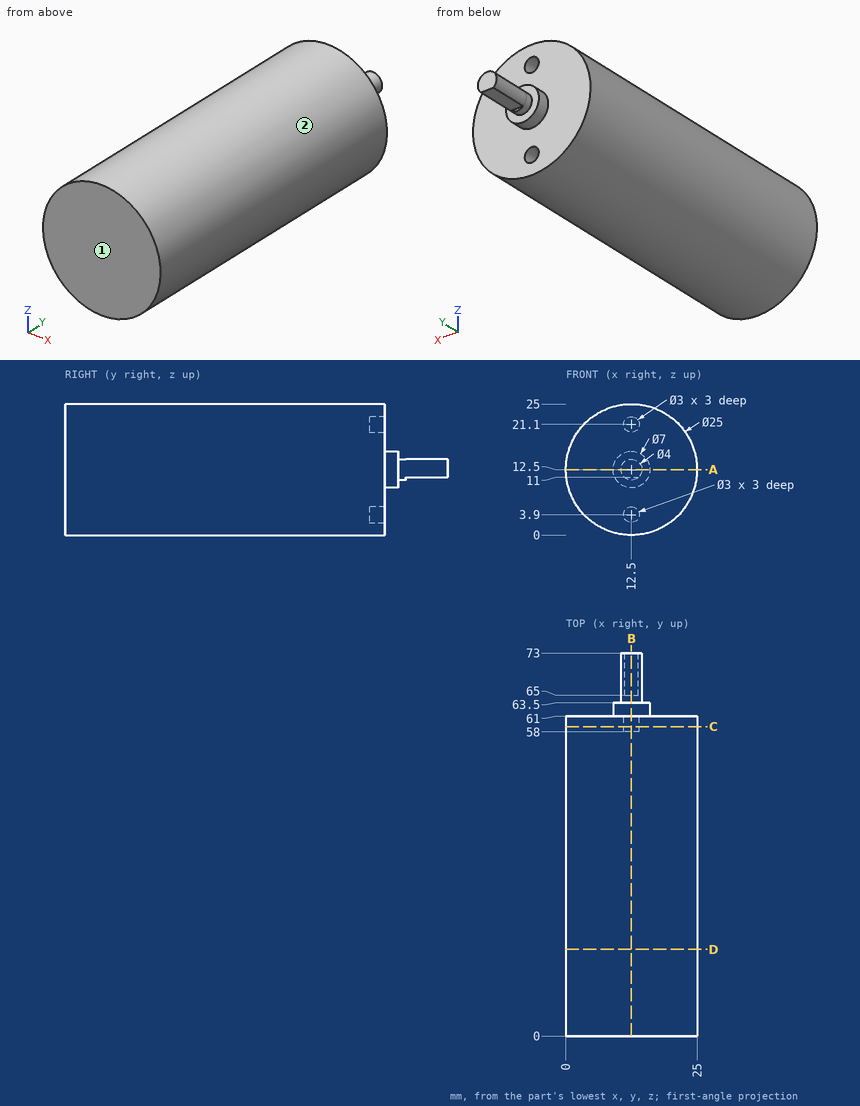
Geometry check sheet. Reference: drawing and pictorial views, mm from the part's lowest x, y, z. Give positions to 0.01 mm unless a question says otherwise; leave off trailing zeros. Loops run counter-clockwise (first coordinate to the right, second up) from the corner with the lowest first, then second, coordinate; pieces in that order, holes last. Notation, with made-up numbers: M 20.5,-1.5 L 34.5,-1.5 A13 cw 34.5,6.5 Z; hole C 37,73 d1. An arc over 180 degrees is marked long. Use a Markdown table: item, result. Add a question column.
Q1. Scan lines: line 1 along Y through (x, z) = (21, 13); line 2 along X through (y, z) = (9, 12.75); line 3 along X through (y, z) = (60.3, 3.9). Record each from-to range of solid material in increasing order. Write a range as [from, to].
Q2. Sectioned sample at C-C, the plane y = 59. Record the cut outline in (x, z).
Q3. Sectioned sample at B-B, the plane x = 12.5. Record the cut outline in (y, z).
Q4. Go/stop test with flat-tipped pins: pin 1 (4 mm diameter, centred on y = 9.5, z = 3.5, fed in from -X); pin 2 (1.5 mm diameter, centred on x = 3.5, y = 45.5, fed in from -Z); pin 3 (0.9 mm diameter, centred on x = 13, z = 3.5, fed in from +Y). Record where each tip stops, or that it passes through.
Q5. Mould release check, pull along X, two halves, no side actions. Record for the marked faces 1 and 2: pulls with the +X half, pulls with the -X half, needs draft (parallel to the pull), parting line crosses it, or undercut.
Q6. Sectioned sample at D-D, the plane y = 16.5. Record the cut outline in (x, z), then the cut area to 3 significant figures.
Q7. Sectioned sample at A-A, the plane z = 12.5. Record the cut outline in (x, y), then the cut area to 3 significant figures.
Verdict:
| question | item | result |
|---|---|---|
| 1 | line 1 | [0, 61] |
| 1 | line 2 | [0, 25] |
| 1 | line 3 | [3.43, 11], [14, 21.57] |
| 2 | outline | C 12.5,12.5 d25; hole C 12.5,3.9 d3; hole C 12.5,21.1 d3 |
| 3 | outline | M 0,0 L 61,0 L 61,2.4 L 58,2.4 L 58,5.4 L 61,5.4 L 61,9 L 63.5,9 L 63.5,10.5 L 65,10.5 L 65,11 L 73,11 L 73,14.5 L 63.5,14.5 L 63.5,16 L 61,16 L 61,19.6 L 58,19.6 L 58,22.6 L 61,22.6 L 61,25 L 0,25 Z |
| 4 | pin 1 | x = 2.14 |
| 4 | pin 2 | z = 3.11 |
| 4 | pin 3 | y = 58 |
| 5 | face 1 | needs draft |
| 5 | face 2 | parting line crosses it |
| 6 | outline | C 12.5,12.5 d25 |
| 6 | area | 491 mm^2 |
| 7 | outline | M 0,0 L 25,0 L 25,61 L 16,61 L 16,63.5 L 14.5,63.5 L 14.5,73 L 10.5,73 L 10.5,63.5 L 9,63.5 L 9,61 L 0,61 Z |
| 7 | area | 1,580 mm^2 |
